Could you check a few things on this drawing? It's one solid part, dimensions in mm from its lowest x, y, z. A direction names the side the tool comes from. Round coordinates to 2 decimals unless told otherwise and drop trailing zeros. Loops run counter-clockwise (first coordinate to the right, second up) from the corner with the lowest first, then second, coordinate; pieces in that order, holes last. Notation, with made-up numbers: (-12.75, -7) -> (8.25, -7) arc R19 cw to (8.25, 15) -> close; hole circle Ø5 at (46, 77). An arc over 180 degrees is marked (long way). Use one line per item in the form item = value. Start each with the question number.
Item 1: I'm going to push flat-ended pins straight in: pin 1 Ø5 at (y, z) = (13, 8) entering from -X; pin 2 Ø7 at (x, y) = (29, 6) entering from -Z; pin 3 Ø2.5 at (y, z) = (11.5, 19.5) entering from +X; pin 4 Ø1.1 at (y, z) = (2, 8) entering from +X. Where does each tip first touch, or does it pass through?
Item 2: If I drill on L1, parallel to Y at x = 29, z = 1.3; L2, parallel to X at y = 21.5, z = 10.5; L3, parallel to X at y = 26, z = 5, over which ranges is the centre line in solid material (lowest first)? Write a range as [from, to].
Item 3: If we section it at C-C (z = 1.5): Write out the boundary of the cut face in (x, y), then the cut area to 3 significant figures.
Item 4: If we section it at A-A (z = 6): Write out the boundary of the cut face in (x, y), then the cut area to 3 significant figures.
Item 5: If we section it at B-B (x = 29): Write out the boundary of the cut face in (y, z).
Item 6: If we section it at D-D (y = 24): Write out the boundary of the cut face in (x, z).
Item 7: For the marked faces 5, 6, 7, 8 and 9, which set-ups out of +Z, -Z, +X, -X, +Y, -Y let a thin tool reach every point of the face, with its end or its side?
Item 8: Thinking about a two-plate mould opening in X: for the marked faces 1, 2, 3 and 4, which applies, released by +X, released by -X, zero draft, split by the parting line, or undercut?
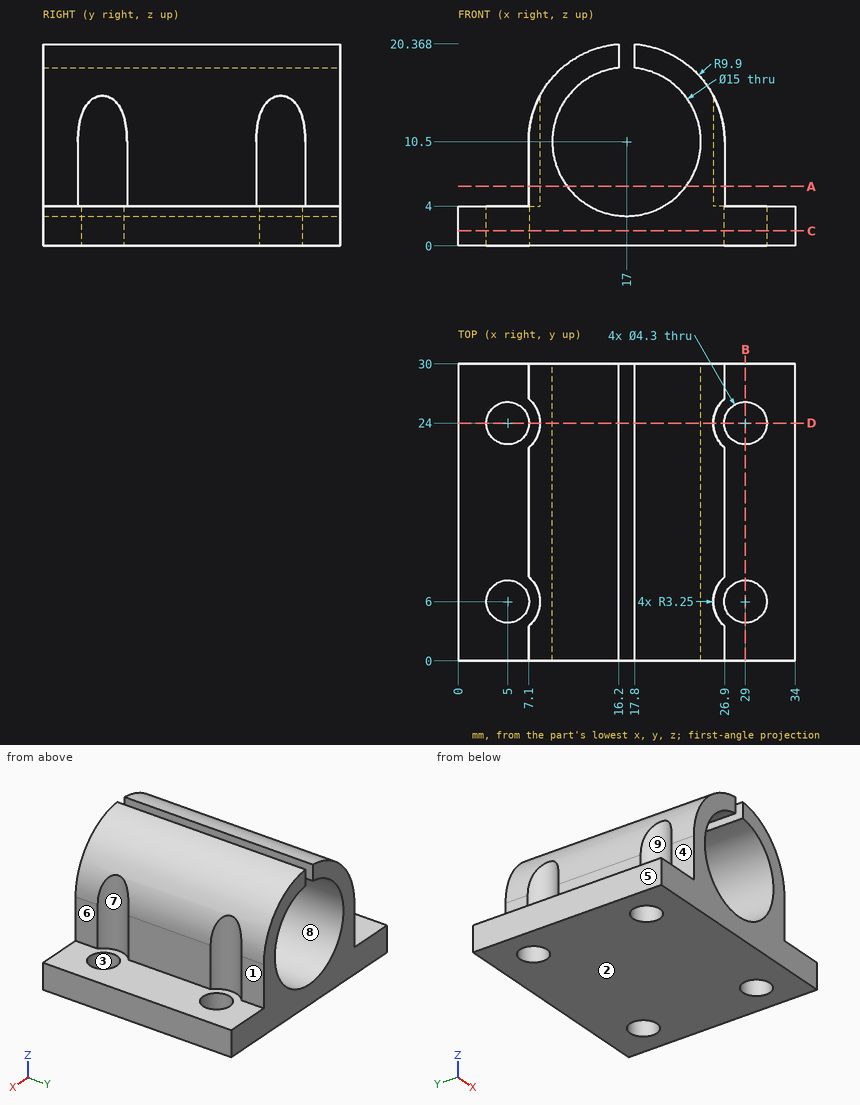
Values found:
q1.pin_1 = 7.1
q1.pin_2 = 0
q1.pin_3 = 23.16
q1.pin_4 = 26.9
q2.L1 = [0, 3.85], [8.15, 21.85], [26.15, 30]
q2.L2 = [7.1, 9.5], [24.5, 26.9]
q2.L3 = [7.56, 11.9], [22.1, 26.44]
q3.outline = (0, 0) -> (34, 0) -> (34, 30) -> (0, 30) -> close; hole circle Ø4.3 at (5, 6); hole circle Ø4.3 at (5, 24); hole circle Ø4.3 at (29, 6); hole circle Ø4.3 at (29, 24)
q3.area = 962 mm2
q4.outline = (7.1, 0) -> (11, 0) -> (11, 30) -> (7.1, 30) -> (7.1, 26.48) arc R3.25 cw to (7.1, 21.52) -> (7.1, 8.48) arc R3.25 cw to (7.1, 3.52) -> close; (23, 0) -> (26.9, 0) -> (26.9, 3.52) arc R3.25 cw to (26.9, 8.48) -> (26.9, 21.52) arc R3.25 cw to (26.9, 26.48) -> (26.9, 30) -> (23, 30) -> close
q4.area = 218 mm2
q5.outline = (0, 0) -> (3.85, 0) -> (3.85, 4) -> (0, 4) -> close; (8.15, 0) -> (21.85, 0) -> (21.85, 4) -> (8.15, 4) -> close; (26.15, 0) -> (30, 0) -> (30, 4) -> (26.15, 4) -> close
q6.outline = (0, 0) -> (2.85, 0) -> (2.85, 4) -> (0, 4) -> close; (7.15, 0) -> (26.85, 0) -> (26.85, 4) -> (25.75, 4) -> (25.75, 15.13) arc R9.9 ccw to (17.8, 20.37) -> (17.8, 17.96) arc R7.5 cw (long way) to (16.2, 17.96) -> (16.2, 20.37) arc R9.9 ccw to (8.25, 15.13) -> (8.25, 4) -> (7.15, 4) -> close; (31.15, 0) -> (34, 0) -> (34, 4) -> (31.15, 4) -> close
q7.face_5 = +Z, -Z, -X, +Y, -Y
q7.face_6 = +Z, +X, +Y, -Y
q7.face_7 = +Z, +X
q7.face_8 = +Y, -Y
q7.face_9 = +Z, -X
q8.face_1 = released by +X
q8.face_2 = zero draft
q8.face_3 = undercut
q8.face_4 = released by -X
